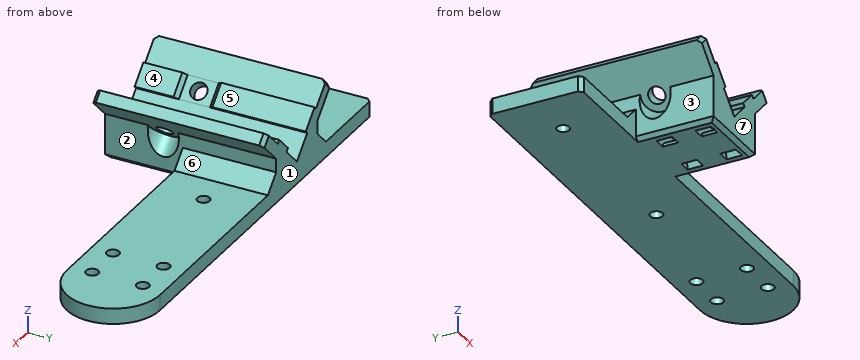
from build123d import *

# Parameters (mm, degrees)
CROQUIS1_R                 = 1.6
SALIENTE_EXTRUIR1_DEPTH    = 4
CROQUIS3_R                 = 1.6
SALIENTE_EXTRUIR3_DEPTH    = 4
SALIENTE_EXTRUIR4_DEPTH    = 44
CORTAR_EXTRUIR1_START      = -2
CORTAR_EXTRUIR1_DEPTH      = 4
MATRIZL1_COUNT             = 2
MATRIZL1_PITCH             = 10
CORTAR_EXTRUIR2_DEPTH      = 86.777797157
CORTAR_EXTRUIR2_DEPTH_BACK = 86.777797157
CROQUIS7_R                 = 2.1
CROQUIS8_R                 = 4
CORTAR_EXTRUIR3_DEPTH      = 86.777797157
CORTAR_EXTRUIR4_DEPTH      = 88.170949948
CORTAR_EXTRUIR4_DEPTH_BACK = 88.170949948
CROQUIS9_R                 = 2.1
CROQUIS10_R                = 4
CORTAR_EXTRUIR5_DEPTH      = 88.170949948
CHAFL_N1_SIZE              = 4
CHAFL_N2_SIZE              = 1
CROQUIS11_W                = 6
CROQUIS11_H                = 8
CORTAR_EXTRUIR6_DEPTH      = 1
CROQUIS12_W                = 6
CROQUIS12_H                = 8
CORTAR_EXTRUIR7_DEPTH      = 1
CHAFL_N3_SIZE              = 1


with BuildPart() as part:
    # Croquis1 → Saliente-Extruir1 (new body)
    with BuildSketch(Plane.XY):
        Polygon((10, -12), (36, -12), (36, 12), (-36, 12), (-36, -12), (-10, -12), (-10, -32), (10, -32), align=None)
        with Locations((-22.5, 0)):
            Circle(CROQUIS1_R, mode=Mode.SUBTRACT)
        with Locations(Location((22.5, 0, 0), (0, 0, 180))):
            Circle(CROQUIS1_R, mode=Mode.SUBTRACT)
    extrude(amount=SALIENTE_EXTRUIR1_DEPTH)

    # Croquis3 → Saliente-Extruir3 (add)
    with BuildSketch(Plane(origin=(0, 0, 0), x_dir=(-1, 0, 0), z_dir=(0, 0, -1))):
        with BuildLine():
            Line((-66, 12), (-36, 12))
            Line((-36, 12), (-36, -12))
            Line((-36, -12), (-66, -12))
            ThreePointArc((-66, -12), (-78, 0), (-66, 12))
        make_face()
        with Locations((-54, 6.5)):
            Circle(CROQUIS3_R, mode=Mode.SUBTRACT)
        with Locations((-64, 6.5)):
            Circle(CROQUIS3_R, mode=Mode.SUBTRACT)
        with Locations(Location((-54, -6.5, 0), (0, 0, 180))):
            Circle(CROQUIS3_R, mode=Mode.SUBTRACT)
        with Locations(Location((-64, -6.5, 0), (0, 0, 180))):
            Circle(CROQUIS3_R, mode=Mode.SUBTRACT)
    extrude(amount=-SALIENTE_EXTRUIR3_DEPTH)

    # Croquis5 → Saliente-Extruir4 (add, through all)
    with BuildSketch(Plane(origin=(0, 12, 0), x_dir=(1, 0, 0), z_dir=(0, 1, 0))):
        Polygon((-10, -11.544513011), (-10, -4), (10, -4), (10, -11.544513011), (16.334166645, -17.878679656), (14.212846302, -20), (9.227743494, -15.014897193), (8.520636713, -15.722003974), (4.277996026, -11.479363287), (4.985102807, -10.772256506), (0, -5.787153698), (-4.985102807, -10.772256506), (-4.277996026, -11.479363287), (-8.520636713, -15.722003974), (-9.227743494, -15.014897193), (-14.212846302, -20), (-16.334166645, -17.878679656), align=None)
    extrude(amount=-SALIENTE_EXTRUIR4_DEPTH)

    # Croquis6 → Cortar-Extruir1 (cut)
    with BuildSketch(Plane.XZ.offset(32).offset(CORTAR_EXTRUIR1_START)):
        with BuildLine():
            Line((-4.48819847, 0), (-7.48819847, 0))
            ThreePointArc((-7.48819847, 0), (-6.174348725, 3.177805305), (-3, 4.499984525))
            Line((-3, 4.499984525), (3, 4.499984525))
            ThreePointArc((3, 4.499984525), (6.174348725, 3.177805305), (7.48819847, 0))
            Line((7.48819847, 0), (4.48819847, 0))
            ThreePointArc((4.48819847, 0), (4.036842813, 1.072541394), (2.954405081, 1.499619287))
            Line((2.954405081, 1.499619287), (-2.954405081, 1.499619287))
            ThreePointArc((-2.954405081, 1.499619287), (-4.036842813, 1.072541394), (-4.48819847, 0))
        make_face()
    cortar_extruir1 = extrude(amount=-CORTAR_EXTRUIR1_DEPTH, mode=Mode.SUBTRACT)

    # MatrizL1: Cortar-Extruir1 ×2
    with Locations(*[(0, i * MATRIZL1_PITCH, 0) for i in range(1, MATRIZL1_COUNT)]):
        add(cortar_extruir1, mode=Mode.SUBTRACT)

    # Croquis7 → Cortar-Extruir2 (cut, two sides: drawn at the far end of the back side and taken through both)
    with BuildSketch(Plane(origin=(0.772256506, 0, 0.772256506), x_dir=(-0.7071067811865476, 0, 0.7071067811865476), z_dir=(-0.7071067811865476, 0, -0.7071067811865476)).offset(-CORTAR_EXTRUIR2_DEPTH_BACK)):
        with Locations(Location((14.142135624, -17, 0), (0, 0, 58.663416321))):
            Circle(CROQUIS7_R)
    extrude(amount=CORTAR_EXTRUIR2_DEPTH + CORTAR_EXTRUIR2_DEPTH_BACK, mode=Mode.SUBTRACT)

    # Croquis8 → Cortar-Extruir3 (cut, through all)
    with BuildSketch(Plane(origin=(0.772256506, 0, 0.772256506), x_dir=(-0.7071067811865476, 0, 0.7071067811865476), z_dir=(-0.7071067811865476, 0, -0.7071067811865476))):
        with Locations((14.142135624, -17)):
            Circle(CROQUIS8_R)
    extrude(amount=CORTAR_EXTRUIR3_DEPTH, mode=Mode.SUBTRACT)

    # Croquis9 → Cortar-Extruir4 (cut, two sides: drawn at the far end of the back side and taken through both)
    with BuildSketch(Plane(origin=(-0.772256506, 0, 0.772256506), x_dir=(-0.7071067811865476, 0, -0.7071067811865476), z_dir=(0.7071067811865476, 0, -0.7071067811865476)).offset(-CORTAR_EXTRUIR4_DEPTH_BACK)):
        with Locations(Location((-14.142135624, -17, 0), (0, 0, 238.663416321))):
            Circle(CROQUIS9_R)
    extrude(amount=CORTAR_EXTRUIR4_DEPTH + CORTAR_EXTRUIR4_DEPTH_BACK, mode=Mode.SUBTRACT)

    # Croquis10 → Cortar-Extruir5 (cut, through all)
    with BuildSketch(Plane(origin=(-0.772256506, 0, 0.772256506), x_dir=(-0.7071067811865476, 0, -0.7071067811865476), z_dir=(0.7071067811865476, 0, -0.7071067811865476))):
        with Locations((-14.142135624, -17)):
            Circle(CROQUIS10_R)
    extrude(amount=CORTAR_EXTRUIR5_DEPTH, mode=Mode.SUBTRACT)

    # Chaflán1
    chafl_n1_edges = [part.edges().sort_by_distance(p)[0] for p in [
        (-10, 0, 4),
        (10, 0, 4),
    ]]
    chamfer(chafl_n1_edges, length=CHAFL_N1_SIZE)

    # Chaflán2
    chafl_n2_edges = [part.edges().sort_by_distance(p)[0] for p in [
        (-36, -12, 2),
        (-36, 12, 2),
        (-15.273506474, -32, 18.939339828),
        (15.273506474, -32, 18.939339828),
        (15.273506474, 12, 18.939339828),
        (-15.273506474, 12, 18.939339828),
        (10, -22, 0),
        (0, -32, 0),
        (-10, -22, 0),
    ]]
    chamfer(chafl_n2_edges, length=CHAFL_N2_SIZE)

    # Croquis11 → Cortar-Extruir6 (cut)
    with BuildSketch(Plane(origin=(-3.60068363, 0, 3.60068363), x_dir=(0.7071067811865476, 0, 0.7071067811865476), z_dir=(-0.7071067811865476, 0, 0.7071067811865476))):
        with Locations((14.142135624, -17)):
            Rectangle(CROQUIS11_W, CROQUIS11_H)
    extrude(amount=-CORTAR_EXTRUIR6_DEPTH, mode=Mode.SUBTRACT)

    # Croquis12 → Cortar-Extruir7 (cut)
    with BuildSketch(Plane(origin=(3.60068363, 0, 3.60068363), x_dir=(0.7071067811865475, 0, -0.7071067811865477), z_dir=(0.7071067811865477, 0, 0.7071067811865475))):
        with Locations((-14.142135624, -17)):
            Rectangle(CROQUIS12_W, CROQUIS12_H)
    extrude(amount=-CORTAR_EXTRUIR7_DEPTH, mode=Mode.SUBTRACT)

    # Chaflán3
    chafl_n3_edges = [part.edges().sort_by_distance(p)[0] for p in [
        (-6.39931637, -21, 13.60068363),
        (6.39931637, -21, 13.60068363),
        (6.39931637, -13, 13.60068363),
        (-6.39931637, -13, 13.60068363),
    ]]
    chamfer(chafl_n3_edges, length=CHAFL_N3_SIZE - 0.0001)  # a hair under: the kernel refuses the full size


solid = part.part
Verification items for the finished model (mm, model axes). Face numbers are marked on the shaded views. A direction names the side the tool comes from. Coordinates: 2 decimals unless noted, no trailing zeros. Order: outer loops, then holes, each group sorted by start corner. A loop starts at its lowest first (then second) coordinate and runs counter-clockwise, first axis right, second up.
Item 1: Depth check by flat-ended pin: pin 1 (4 mm diameter, centred on x = 51, z = 3, fed in from -Y); pin 2 (8 mm diameter, centred on y = 2.5, z = 8.5, fed in from +X); pin 3 (10 mm diameter, centred on y = -9.5, z = 16.5, fed in from +X). Enter the tip coordinate at first touch or a pass-through.
Filled in:
pin 1: stops at y = -12
pin 2: stops at x = 13.5
pin 3: stops at x = 16.33
Item 2: Section check A-A, the plane x = -22.5. Enter the section's corners in (y, z).
Filled in:
outline: (-12, 0) - (-1.6, 0) - (-1.6, 4) - (-12, 4) - close; (1.6, 0) - (12, 0) - (12, 4) - (1.6, 4) - close
Item 3: Material ranges on L1, parallel to Y at x = 64, z = 2.6; L2, parallel to Y at x = -1.5, z = 2; L3, parallel to Y at x = -22.5, z = 3, recorded low to high.
Filled in:
L1: y = -12 to -8.1, -4.9 to 4.9, 8.1 to 12
L2: y = -32 to -30, -26 to -20, -16 to 12
L3: y = -12 to -1.6, 1.6 to 12
Item 4: Section check D-D, the plane y = -25. Enter the section's corners in (x, z), then the cut area to 3 significant figures.
Filled in:
outline: (-16.33, 17.88) - (-10, 11.54) - (-10, 1) - (-9, 0) - (9, 0) - (10, 1) - (10, 11.54) - (16.33, 17.88) - (14.21, 20) - (9.23, 15.01) - (8.52, 15.72) - (4.28, 11.48) - (4.99, 10.77) - (0, 5.79) - (-4.99, 10.77) - (-4.28, 11.48) - (-8.52, 15.72) - (-9.23, 15.01) - (-14.21, 20) - close
area: 271 mm2
Item 5: Access from +Z, -Z, +X, -X, +Y, -Y to the whole of each face (thin tool, end or side, straight path). Record for the marked faces 1, 2, 3 and 4.
Filled in:
face 1: +Z, -Z, +X, -X, +Y
face 2: +X, -Y
face 3: -X, -Y
face 4: +Z, +Y, -Y
Item 6: Release check for a two-part mould opening along Z. For the marked faces 5, 6 and 7 record: +Z half, -Z half, draft (parallel to the pull), parting line (faces both ways), or undercut.
Filled in:
face 5: +Z half
face 6: undercut
face 7: draft
Item 7: Section check C-C, the plane x = 54. Enter the section's corners in (y, z).
Filled in:
outline: (-12, 0) - (-8.1, 0) - (-8.1, 4) - (-12, 4) - close; (-4.9, 0) - (4.9, 0) - (4.9, 4) - (-4.9, 4) - close; (8.1, 0) - (12, 0) - (12, 4) - (8.1, 4) - close
Item 8: Section check B-B, the plane y = 0. Give the number of separate pieces and of enclosed holes in the cut face, then the cut area to 3 significant figures.
Filled in:
separate pieces: 3
enclosed holes: 0
area: 639 mm2
